Read the model definition and answer for the solid it produces. Units are mm, in the model's axes. A direction names the side the tool comes from. Coordinates: 2 decimals unless noted, no trailing zeros. Write each loop counter-clockwise with the first axis right and the second up, starting at its lowest first coordinate (ties: lowest second). Pieces come first, ordered by that corner, then holes. Notation, with made-up numbers: (83.25, 28.5) -> (125.25, 28.5) arc R15 cw to (125.25, 45.5) -> close; hole circle Ø8 at (67.5, 7.5). An arc over 180 degrees is marked (long way). Answer as a JSON object with one key per item and string values. Group by question number.
(1) For a pull along Y with two mould halves and no side action, classify faces 5 (the face through (11, -21.542, -25)), 6 (the face through (33.764, -51, -35)), 7 (the face through (-1.6, -37, -35)) as +Y half, -Y half, draft (parallel to the pull), parting line (faces both ways), or undercut.
(2) Which of the six approach directions +Z, -Z, +X, -X, +Y, -Y give full straight-line access (tool end or side, diameter ignored) to faces 1 (the face through (11, 2, 0)), 2 (the face through (17, -49.642, -35)), 3 (the face through (20.605, -51.251, -35.036)), 4 (the face through (0, -8, 1))?
(3) Flat-ended cylindrical pins translate along their axes: P1, Ø12, axis at x = 14.5, z = -37.5, coming from the +Y side; P2, Ø11, axis at x = 14, y = 7, coming from the -Z side; P3, Ø17.5, axis at y = -38.5, z = -35, coming from the +X side; P4, Ø12, axis at x = 28.5, y = 6, coming from the +Z side. Find the tip coordinate at first contact, or state that the pin passes through.
(4) Find section C-C (x = 12). Give the vertices of the cut face in (y, z) (3 decimals), then the cut area to 3 significant figures.
(5) Find section B-B (z = -27). Give the vertices of the cut face in (x, y) (3 decimals).
(6) Straight lines are drawn through the part: L1, parallel to Y at x = 18, z = -44; L2, parallel to Y at x = 1.5, z = -13; L3, parallel to X at y = -30.5, z = -39.5 (3 decimals). For each, find the intervals that lie inside material, in ascending order.
(7) Find section A-A (x = 16). Give the vertices of the cut face in (y, z) (3 decimals).
(8) Find section D-D (y = -37). Give the vertices of the cut face in (x, z) (3 decimals).
from build123d import *

# Parameters (mm, degrees)
SKETCH1_W                    = 21.59
SKETCH1_H                    = 43.18
SKETCH1_R                    = 4.124999878
BOSS_EXTRUDE1_DEPTH          = 3.175
EDGE_FLANGE1_STRIP_W         = 19.05
EDGE_FLANGE1_STRIP_H         = 3.175
EDGE_FLANGE1_STRIP_CUT_DEPTH = 21.59
EDGE_FLANGE1_DEPTH           = 21.59
EDGE_FLANGE2_DEPTH           = 22.48154
EDGE_FLANGE2_START           = 3.175
EDGE_FLANGE2_FLAT_DEPTH      = 3.175
EDGE_FLANGE3_STRIP_W         = 15.900000204
EDGE_FLANGE3_STRIP_H         = 3.175
EDGE_FLANGE3_STRIP_CUT_DEPTH = 22.48154
EDGE_FLANGE3_DEPTH           = 22.48154
CUT_EXTRUDE2_REACH           = 96.019
SKETCH11_R                   = 3.57124


# Sheet-metal steps are written as plain solids
with BuildPart() as part:
    # Sketch1 → Boss-Extrude1 (new body)
    with BuildSketch(Plane.XY):
        with Locations((10.795, 0.048317484)):
            Rectangle(SKETCH1_W, SKETCH1_H)
        with Locations(Location((10.795, 11.418627484, 0), (0, 0, 180))):
            Circle(SKETCH1_R, mode=Mode.SUBTRACT)
    extrude(amount=BOSS_EXTRUDE1_DEPTH)

    # Edge-Flange1 strip (across the edge) → Edge-Flange1 strip cut (cut)
    with BuildSketch(Plane(origin=(21.59, -21.541682516, 0), x_dir=(0, 1, 0), z_dir=(-1, 0, 0))):
        with Locations((-6.35, -1.5875)):
            Rectangle(EDGE_FLANGE1_STRIP_W, EDGE_FLANGE1_STRIP_H)
    extrude(amount=EDGE_FLANGE1_STRIP_CUT_DEPTH, mode=Mode.SUBTRACT)

    # Edge-Flange1 section (across the edge) → Edge-Flange1 (add)
    with BuildSketch(Plane(origin=(21.59, -21.541682516, 0), x_dir=(0, 1, 0), z_dir=(-1, 0, 0))):
        with BuildLine():
            Line((-3.175, 3.175), (-3.175, 46.43374))
            Line((-3.175, 46.43374), (0, 46.43374))
            Line((0, 46.43374), (0, 3.175))
            ThreePointArc((0, 3.175), (0.92993597, 0.92993597), (3.175, 0))
            Line((3.175, 0), (3.175, -3.175))
            ThreePointArc((3.175, -3.175), (-1.315128061, -1.315128061), (-3.175, 3.175))
        make_face()
    extrude(amount=EDGE_FLANGE1_DEPTH)

    # Edge-Flange2 bend section (across the edge) → Edge-Flange2 (add)
    with BuildSketch(Plane(origin=(-1.600000102, -24.716682516, -23.9522), x_dir=(1, 0, 0), z_dir=(0, 0, -1))):
        with BuildLine():
            Line((-3.175, 1.600000102), (0, 1.600000102))
            ThreePointArc((0, 1.600000102), (0.46862918, 0.46862918), (1.600000102, 0))
            Line((1.600000102, 0), (1.600000102, -3.175))
            ThreePointArc((1.600000102, -3.175), (-1.77643485, -1.77643485), (-3.175, 1.600000102))
        make_face()
    extrude(amount=EDGE_FLANGE2_DEPTH)

    # Edge-Flange2 profile (on flange) → Edge-Flange2 flat (add)
    with BuildSketch(Plane(origin=(-1.600000102, -24.716682516, 0), x_dir=(0, 0, -1), z_dir=(-1, 0, 0)).offset(EDGE_FLANGE2_START)):
        Polygon((23.9522, 28.10002), (23.9522, 19.3675), (23.9522, 1.600000102), (46.43374, 1.600000102), (46.43374, 28.10002), align=None)
    extrude(amount=-EDGE_FLANGE2_FLAT_DEPTH)

    # Edge-Flange3 strip (across the edge) → Edge-Flange3 strip cut (cut)
    with BuildSketch(Plane(origin=(-1.600000102, -52.816702516, -23.9522), x_dir=(0, 1, 0), z_dir=(0, 0, -1))):
        with Locations((-3.175, -1.5875)):
            Rectangle(EDGE_FLANGE3_STRIP_W, EDGE_FLANGE3_STRIP_H)
    extrude(amount=EDGE_FLANGE3_STRIP_CUT_DEPTH, mode=Mode.SUBTRACT)

    # Edge-Flange3 section (across the edge) → Edge-Flange3 (add)
    with BuildSketch(Plane(origin=(-1.600000102, -52.816702516, -23.9522), x_dir=(0, 1, 0), z_dir=(0, 0, -1))):
        with BuildLine():
            Line((0, 1.600000102), (0, 35.364220102))
            Line((0, 35.364220102), (3.175, 35.364220102))
            Line((3.175, 35.364220102), (3.175, 1.600000102))
            ThreePointArc((3.175, 1.600000102), (3.64362918, 0.46862918), (4.775000102, 0))
            Line((4.775000102, 0), (4.775000102, -3.175))
            ThreePointArc((4.775000102, -3.175), (1.39856515, -1.77643485), (0, 1.600000102))
        make_face()
    extrude(amount=EDGE_FLANGE3_DEPTH)

    # Sketch11 → Cut-Extrude2 (cut, up to next)
    with BuildSketch(Plane.XZ.offset(52.816702516), mode=Mode.PRIVATE) as cut_extrude2_sk1:
        with Locations((24.17318, -35.19297)):
            Circle(SKETCH11_R)
    cut_extrude2_tool1 = extrude(cut_extrude2_sk1.sketch, amount=-CUT_EXTRUDE2_REACH, mode=Mode.PRIVATE) & part.part
    add(cut_extrude2_tool1.solids().sort_by_distance((24.17318, -52.816703, -35.19297))[0], mode=Mode.SUBTRACT)


solid = part.part
Results below:
{
 "1": {"face 5": "+Y half", "face 6": "draft", "face 7": "undercut"},
 "2": {"face 1": "-Z, +X, -X, +Y", "face 2": "+Z, -Z, +X", "face 3": "-Y", "face 4": "+Z, -X, +Y, -Y"},
 "3": {"P1": "stops at y = -21.54", "P2": "stops at z = 0", "P3": "stops at x = -1.6", "P4": "passes through"},
 "4": {"outline": "(-52.817, -46.434) -> (-49.642, -46.434) -> (-49.642, -23.952) -> (-52.817, -23.952) -> close; (-24.717, -46.434) -> (-21.542, -46.434) -> (-21.542, -3.175) arc R3.175 cw to (-18.367, 0) -> (7.474, 0) -> (7.474, 3.175) -> (-18.367, 3.175) arc R6.35 ccw to (-24.717, -3.175) -> close; (15.364, 0) -> (21.638, 0) -> (21.638, 3.175) -> (15.364, 3.175) -> close", "area": "334 mm2"},
 "5": {"outline": "(-4.775, -48.042) arc R4.775 ccw to (0, -52.817) -> (33.764, -52.817) -> (33.764, -49.642) -> (0, -49.642) arc R1.6 cw to (-1.6, -48.042) -> (-1.6, -26.317) arc R1.6 cw to (0, -24.717) -> (21.59, -24.717) -> (21.59, -21.542) -> (0, -21.542) arc R4.775 ccw to (-4.775, -26.317) -> close"},
 "6": {"L1": "y = -52.82 to -49.64, -24.72 to -21.54", "L2": "y = -24.72 to -21.54", "L3": "x = -4.775 to -1.6"},
 "7": {"outline": "(-52.817, -46.434) -> (-49.642, -46.434) -> (-49.642, -23.952) -> (-52.817, -23.952) -> close; (-24.717, -46.434) -> (-21.542, -46.434) -> (-21.542, -3.175) arc R3.175 cw to (-18.367, 0) -> (21.638, 0) -> (21.638, 3.175) -> (-18.367, 3.175) arc R6.35 ccw to (-24.717, -3.175) -> close"},
 "8": {"outline": "(-4.775, -46.434) -> (-1.6, -46.434) -> (-1.6, -23.952) -> (-4.775, -23.952) -> close"}
}
